```python
from build123d import *

# Parameters (mm, degrees)
SKETCH017_W     = 9.99
SKETCH017_H     = 27.5
PAD007_DEPTH    = 76.2
SKETCH018_R     = 6
POCKET005_DEPTH = 38.326
FILLET003_R     = 1
FILLET004_R     = 1


with BuildPart() as part:
    # Sketch016 → Revolution004 (revolve)
    with BuildSketch(Plane.YZ):
        with BuildLine():
            Line((0, 40), (33.33, 40))
            Line((33.33, 40), (33.33, 20))
            ThreePointArc((33.33, 20), (32.183058, 10.029219), (31.8, 0))
            Line((31.8, 0), (0, 0))
            Line((0, 40), (0, 0))
        make_face()
    revolve(axis=Axis((0, 0, 0), (0, 0, 1)))

    # Sketch017 (on Face1 of Revolution004) → Pad007 (new body)
    with BuildSketch(Plane(origin=(0, 0, 40), x_dir=(0, -1, 0), z_dir=(0, 0, 1))):
        Rectangle(SKETCH017_W, SKETCH017_H)
    extrude(amount=PAD007_DEPTH)

    # Sketch018 (on Face5 of Pad007) → Pocket005 (cut, through all)
    with BuildSketch(Plane(origin=(0, -4.995, 0), x_dir=(0, 0, -1), z_dir=(0, -1, 0))):
        with Locations((-106.2, 0)):
            Circle(SKETCH018_R)
    extrude(amount=-POCKET005_DEPTH, mode=Mode.SUBTRACT)

    # Fillet003
    fillet003_edges = [part.edges().sort_by_distance(p)[0] for p in [
        (0, 4.995, 116.2),
        (-13.75, 0, 116.2),
        (0, -4.995, 116.2),
        (13.75, 0, 116.2),
        (13.75, -4.995, 78.1),
        (13.75, 4.995, 78.1),
        (-13.75, 4.995, 78.1),
        (-13.75, -4.995, 78.1),
    ]]
    fillet(fillet003_edges, radius=FILLET003_R)

    # Fillet004
    fillet004_edges = [part.edges().sort_by_distance(p)[0] for p in [
        (0, -33.33, 20),
        (0, -31.8, 0),
    ]]
    fillet(fillet004_edges, radius=FILLET004_R)


solid = part.part
```
Here's how the part is built. I have some questions about the finished solid (model axes, mm). A direction names the side the tool comes from. Coordinates: 2 decimals unless noted, no trailing zeros. Order: outer loops, then holes, each group sorted by start corner. A loop starts at its lowest first (then second) coordinate and runs counter-clockwise, first axis right, second up. Notation, with made-up numbers: (40, 5) -> (46, 5) arc R24 cw to (46, 38) -> close; hole circle Ø7 at (2.25, 21). An arc over 180 degrees is marked (long way). Return JSON: item names as keys, results as strings.
1) Thinking about a two-plate mould opening in Z: for faces 1 (the flat face through (0, 0, 0)), 2 (the flat face through (13.75, 0, 77)), 3 (the cylindrical face through (1.802, -0.07, 100.477)), which applies, +Z half, -Z half, draft (parallel to the pull), parting line (faces both ways), or undercut?
Conclusion:
{"face 1": "-Z half", "face 2": "draft", "face 3": "undercut"}
2) On a 3-axis mill with a long thin cutter (end or side, diameter ignored), from which of +Z, -Z, +X, -X, +Y, -Y can I reach the whole of each face in a straight line? I mean faces 4 (the flat face through (0, 4.995, 77)), 5 (the cylindrical face through (-10.01, 31.79, 29.9)), 6 (the flat face through (0, 0, 116.2)), 7 (the flat face through (-13.75, 0, 77)), 8 (the flat face through (0, -4.995, 77)). Say none if no direction works.
Conclusion:
{"face 4": "+Z, +X, -X, +Y", "face 5": "+Z, -Z", "face 6": "+Z, +X, -X, +Y, -Y", "face 7": "+Z, -X, +Y, -Y", "face 8": "+Z, +X, -X, -Y"}
3) If I drill on probe 1 along X at (y, z) = (2.75, 106.2); probe 2 along Z at (x, y) = (-12, 20); probe 3 along X at (y, z) = (0.5, 73), over which ranges is the centre line in solid material (lowest first)?
Conclusion:
{"probe 1": "x = -13.75 to -6, 6 to 13.75", "probe 2": "z = 0 to 40", "probe 3": "x = -13.75 to 13.75"}
4) If we section it at B-B on z = 42.5: List the corners of the cut face in (x, y) for me (3 decimals), plus the area to 3 significant figures.
Conclusion:
{"outline": "(-13.75, -3.995) arc R1 ccw to (-12.75, -4.995) -> (12.75, -4.995) arc R1 ccw to (13.75, -3.995) -> (13.75, 3.995) arc R1 ccw to (12.75, 4.995) -> (-12.75, 4.995) arc R1 ccw to (-13.75, 3.995) -> close", "area": "274 mm²"}
5) I'm going to push flat-ended pins straight in: P1, Ø6, axis at x = 26, y = -23.5, coming from the +Z side; P2, Ø6.5, axis at y = 1, z = 79, coming from the +X side; P3, Ø3, axis at x = -0.5, z = 103, coming from the +Y side; P4, Ø3, axis at x = -1.5, z = 61, coming from the -Y side (3 decimals). Where does each tip first touch, or does it pass through?
Conclusion:
{"P1": "stops at z = 40", "P2": "stops at x = 13.75", "P3": "passes through", "P4": "stops at y = -4.995"}
6) If we section it at A-A on z = 106.2: List the corners of the cut face in (x, y) for me (3 decimals), plus the area to 3 significant figures.
Conclusion:
{"outline": "(-13.75, -3.995) arc R1 ccw to (-12.75, -4.995) -> (-6, -4.995) -> (-6, 4.995) -> (-12.75, 4.995) arc R1 ccw to (-13.75, 3.995) -> close; (6, -4.995) -> (12.75, -4.995) arc R1 ccw to (13.75, -3.995) -> (13.75, 3.995) arc R1 ccw to (12.75, 4.995) -> (6, 4.995) -> close", "area": "154 mm²"}
